Autodesk Inventor part; units mm, degrees
ref_plane "YZ Plane" through (0, 0, 0) normal (1, 0, 0) x (0, 1, 0)
ref_plane "XZ Plane" through (0, 0, 0) normal (0, 1, 0) x (-1, 0, 0)
ref_plane "XY Plane" through (0, 0, 0) normal (0, 0, 1) x (1, 0, 0)
sketch "Sketch2" plane through (0, 0, 0) normal (0, 1, 0) x (-1, 0, 0)
  line L0 (-22, 59.152) -> (-34, 59.152)
  arc A0 (-34, 59.152) -> (-35.5236, 58.7363) centre (-34, 56.152) ccw
  arc A1 (-35.5236, 58.7363) -> (-36.5843, 57.6756) centre (-34, 56.152) ccw
  arc A2 (-36.5843, 57.6756) -> (-37, 56.152) centre (-34, 56.152) ccw
  line L1 (-37, 56.152) -> (-37, 44.152)
  arc A3 (-37, 44.052) -> (-34, 41.052) centre (-34, 44.052) ccw
  line L2 (-33.9, 41.052) -> (-21.9, 41.052)
  arc A4 (-21.9, 41.052) -> (-18.9, 44.052) centre (-21.9, 44.052) ccw
  line L3 (-18.9, 44.152) -> (-18.9, 56.152)
  arc A5 (-18.9, 56.152) -> (-21.9, 59.152) centre (-21.9, 56.152) ccw
  line L4 (-15.9, 62.152) -> (-40, 62.152)
  line L5 (-40, 62.152) -> (-40, 38.052)
  line L6 (-40, 38.052) -> (-15.9, 38.052)
  line L7 (-15.9, 38.052) -> (-15.9, 62.152)
  line L8 (-21.9, 59.152) -> (-22, 59.152)
  line L9 (-37, 44.152) -> (-37, 44.052)
  line L10 (-33.9, 41.052) -> (-34, 41.052)
  line L11 (-18.9, 44.152) -> (-18.9, 44.052)
  point P0 (0, 0)
  dimension "d6" = 18.1
  dimension "d7" = 18.1
  dimension "d14" = 3
  dimension "d24" = 3
  dimension "d25" = 3
  dimension "d28" = 3
  dimension "d29" = 3
extrude "Extrusion1" add sketch "Sketch2" along normal blind 2
equation "\"BendRadius\" = Thickness"
equation "\"BendReliefWidth\" = Thickness"
equation "\"BendReliefDepth\" = 0.5 * Thickness"
equation "\"CornerReliefSize\" = 4 * Thickness"
equation "\"MinimumRemnant\" = 2 * Thickness"
equation "\"TransitionRadius\" = BendRadius"
equation "\"JacobiRadiusSize\" = BendRadius"
equation "\"GapSize\" = Thickness"
properties part number "mould"
Can you work these out from the model? Positions are in its coordinate system, mm. A direction names the side the tool comes from. Coordinates: 2 decimals unless noted, no trailing zeros. Loops run counter-clockwise (first coordinate to the right, second up) from the corner with the lowest first, then second, coordinate; pieces in that order, holes last. Notation, with made-up numbers: (71, 77) - (125, 77) arc R35 cw to (125, 109) - close; hole circle Ø6 at (39, 70). An arc over 180 degrees is marked (long way). Answer as CSV lines item,"result". Start each with the question number.
1) Thinking about a two-plate mould opening in Z: for faces 1 (the flat face through (40, 1, 50)), 2 (the flat face through (28, 1, 62.152)), 3 (the cylindrical face through (36.897, 0.986, 56.931)), which applies, pulls with the +Z half, pulls with the -Z half, needs draft (parallel to the pull), parting line crosses it, or undercut?
2) I need wall thicknesses on line 1 (X direction, y = 1, z = 55.5); line 2 (Z direction, x = 22.5, y = 0.9); line 3 (X direction, y = 1.4, z = 43). Which ranges of each line are inside material? Lowest first, please. Write a range as from..to.
3) Which directions (+Z, -Z, +X, -X, +Y, -Y) give clear straight access to the entire face, cutting with the end or side of a thin tool? Please do faces 4 (the cylindrical face through (34.8, 0.986, 59.043)), 5 (the flat face through (28, 1, 38.052)).
4) Suppose I cut it at C-C (z = 50.5). Please give me the cut outline in (x, y), plus the area to 3 significant figures.
5) Suppose I cut it at A-A (y = 1.15). Please give me the cut outline in (x, z).
6) Suppose I cut it at B-B (x = 25.5). Please give me the cut outline in (y, z).
7) For pin 1 (10 mm diameter, centred on x = 30, z = 44.5, fed in from +Y), with a flat end and sliding along its axis, tell me the tip position at first contact or that it passes through.
Check result:
1,face 1,"needs draft"
1,face 2,"pulls with the +Z half"
1,face 3,"undercut"
2,line 1,"x = 15.9..18.9, 37..40"
2,line 2,"z = 38.05..41.05, 59.15..62.15"
2,line 3,"x = 15.9..19.09, 36.81..40"
3,face 4,"+Y, -Y"
3,face 5,"-Z, +X, -X, +Y, -Y"
4,outline,"(15.9, 0) - (18.9, 0) - (18.9, 2) - (15.9, 2) - close; (37, 0) - (40, 0) - (40, 2) - (37, 2) - close"
4,area,"12.0 mm²"
5,outline,"(15.9, 38.05) - (40, 38.05) - (40, 62.15) - (15.9, 62.15) - close; hole (18.9, 44.05) arc R3 ccw to (21.9, 41.05) - (34, 41.05) arc R3 ccw to (37, 44.05) - (37, 56.15) arc R3 ccw to (36.58, 57.68) arc R3 ccw to (35.52, 58.74) arc R3 ccw to (34, 59.15) - (21.9, 59.15) arc R3 ccw to (18.9, 56.15) - close"
6,outline,"(0, 38.05) - (2, 38.05) - (2, 41.05) - (0, 41.05) - close; (0, 59.15) - (2, 59.15) - (2, 62.15) - (0, 62.15) - close"
7,pin 1,"stops at y = 2"
